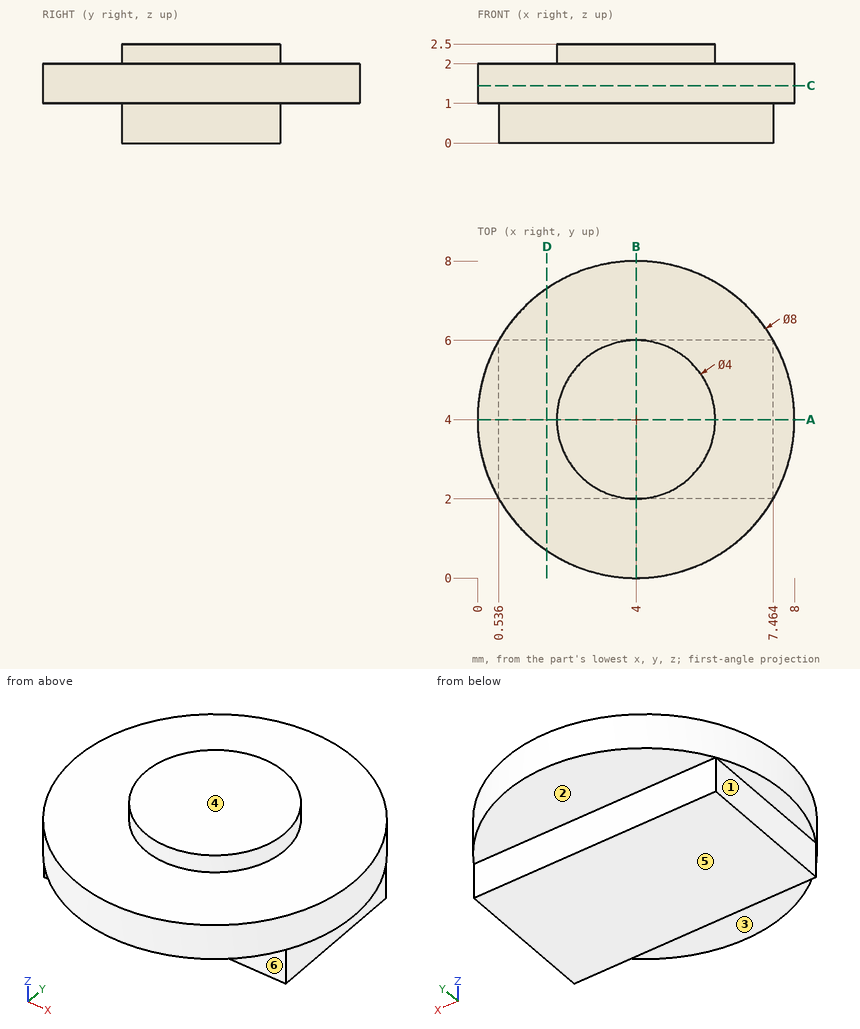
For this review, use the dimensioned drawing (mm, ordinates from the lowest corner) and the shaded views. A direction names the side the tool comes from. Give positions to 0.01 mm unless a question says otherwise; leave off trailing zeros. Write each loop counter-clockwise with the first axis right and the second up, starting at its lowest first coordinate (ties: lowest second). Pieces come first, ordered by that corner, then holes.
(1) To check wall thickness, follow L1, parallel to Z at x = 3.5, y = 1; L2, parallel to Y at x = 3.25, z = 0.9; L3, parallel to X at y = 5.5, z = 0.35. State the ranges of each line that lie inside material, in increasing order.
(2) For P1, Ø0.6, axis at x = 4.5, y = 7, coming from the -Z side; P2, Ø0.5, axis at x = 3, z = 0.5, coming from the +Y side; P3, Ø1.1, axis at y = 3, z = 0.5, coming from the +X side (3 decimals), all flat-tipped, find the tip position at first contact; note any pin that passes through.
(3) Consider section C-C, the plane z = 1.45. Give the boundary of the cut face in (x, y), and give its area (3 significant figures).
(4) Consider section B-B, the plane x = 4. Give the boundary of the cut face in (y, z), and give its area (3 significant figures).
(5) The part is to be moulded in two halves that separate along Z. For the marked faces 4, 5 and 6, say which applies: released by +Z, released by -Z, zero draft, split by the parting line, or undercut.
(6) Consider section A-A, the plane y = 4. Give the boundary of the cut face in (x, z), and give its area (3 significant figures).
(7) Tool access review of the marked faces 1, 2 and 3: name each direction out of +Z, -Z, +X, -X, +Y, -Y from which nothing blocks a thin tool from reaching the whole face with its end or side.
(8) Consider section D-D, the plane x = 1.75. Give the boundary of the cut face in (y, z).
Returned:
1. L1: z = 1 to 2
1. L2: y = 2 to 6
1. L3: x = 0.54 to 7.46
2. P1: stops at z = 1
2. P2: stops at y = 6
2. P3: stops at x = 7.925
3. outline: circle Ø8 at (4, 4)
3. area: 50.3 mm2
4. outline: (0, 1) - (2, 1) - (2, 0) - (6, 0) - (6, 1) - (8, 1) - (8, 2) - (6, 2) - (6, 2.5) - (2, 2.5) - (2, 2) - (0, 2) - close
4. area: 14.0 mm2
5. face 4: released by +Z
5. face 5: released by -Z
5. face 6: zero draft
6. outline: (0, 1) - (0.54, 1) - (0.54, 0) - (7.46, 0) - (7.46, 1) - (8, 1) - (8, 2) - (6, 2) - (6, 2.5) - (2, 2.5) - (2, 2) - (0, 2) - close
6. area: 16.9 mm2
7. face 1: -Z, -X, +Y, -Y
7. face 2: -Z, +X, -X, +Y
7. face 3: -Z, +X, -X, -Y
8. outline: (0.69, 1) - (2, 1) - (2, 0) - (6, 0) - (6, 1) - (7.31, 1) - (7.31, 2) - (0.69, 2) - close
